Build history of the part. All positions in model axes, mm. Face numbers are marked on the shaded views. A direction names the side the tool comes from. Round coordinates to 2 decimals unless told otherwise and drop trailing zeros. Write each loop counter-clockwise with the first axis right and the second up, starting at its lowest first coordinate (ties: lowest second). Pieces come first, ordered by that corner, then holes.
1) Saw through at A-A (y = 97.5). Write the cut outline in (x, z).
2) Flat gauge pins, fed straight in: pin 1 (1.5 mm diameter, centred on x = 5.5, z = 10.5, fed in from -Y); pin 2 (2 mm diameter, centred on x = -6, y = 47.5, fed in from +Z); pin 3 (6 mm diameter, centred on x = 6, y = 79, fed in from -Z). Where does each tip first touch, or does it go through?
3) Wall check: probe 1 along Y at (x, z) = (3.5, -1.5); probe 2 along Y at (x, z) = (7.25, 1.5); probe 3 along X at (y, z) = (10.5, 7.25). Give the ranges that are in metal, low to high.
4) Pull direction Y, two halves, no side cores. Call the marked faces 3 and 4: +Y half, -Y half, draft (parallel to the pull), parting line (faces both ways), or undercut.
5) Which spindle directions (+Z, -Z, +X, -X, +Y, -Y) get a long thin tool onto all of the face, cutting with end or side? Do the marked faces 1 and 2. Say none if no direction does.
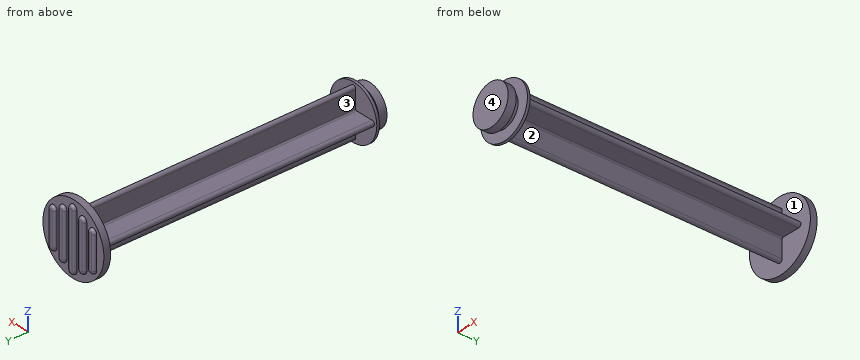
from build123d import *

# Parameters (mm, degrees)
BOSS_EXTRUDE1_DEPTH = 102
SKETCH3_R           = 13
BOSS_EXTRUDE2_DEPTH = 2.5
BOSS_EXTRUDE3_DEPTH = 1
FILLET1_R           = 1


with BuildPart() as part:
    # Sketch1 → Revolve1 (revolve)
    with BuildSketch(Plane.XY, mode=Mode.PRIVATE) as revolve1_sk:
        Polygon((0, 0), (7.5, 0), (7.5, 3), (6, 3), (6, 5), (10, 5), (10, 6), (0, 6), align=None)
    revolve(revolve1_sk.sketch.rotate(Axis((0, 6, 0), (0, -1, 0)), 180), axis=Axis((0, 6, 0), (0, -1, 0)))

    # Sketch2 → Boss-Extrude1 (add)
    with BuildSketch(Plane(origin=(0, 6, 0), x_dir=(1, 0, 0), z_dir=(0, 1, 0))):
        with BuildLine():
            Line((-1, 8), (-1, 1.5))
            ThreePointArc((-1, 1.5), (-1.146446609, 1.146446609), (-1.5, 1))
            Line((-1.5, 1), (-8, 1))
            ThreePointArc((-8, 1), (-9, 0), (-8, -1))
            Line((-8, -1), (-1.5, -1))
            ThreePointArc((-1.5, -1), (-1.146446609, -1.146446609), (-1, -1.5))
            Line((-1, -1.5), (-1, -8))
            ThreePointArc((-1, -8), (0, -9), (1, -8))
            Line((1, -8), (1, -1.5))
            ThreePointArc((1, -1.5), (1.146446609, -1.146446609), (1.5, -1))
            Line((1.5, -1), (8, -1))
            ThreePointArc((8, -1), (9, 0), (8, 1))
            Line((8, 1), (1.5, 1))
            ThreePointArc((1.5, 1), (1.146446609, 1.146446609), (1, 1.5))
            Line((1, 1.5), (1, 8))
            ThreePointArc((1, 8), (0, 9), (-1, 8))
        make_face()
    extrude(amount=BOSS_EXTRUDE1_DEPTH)

    # Sketch3 → Boss-Extrude2 (add)
    with BuildSketch(Plane(origin=(0, 108, 0), x_dir=(1, 0, 0), z_dir=(0, 1, 0))):
        with Locations(Location((0, 0, 0), (0, 0, 180))):
            Circle(SKETCH3_R)
    extrude(amount=BOSS_EXTRUDE2_DEPTH)

    # Sketch4 → Boss-Extrude3 (add)
    with BuildSketch(Plane(origin=(0, 110.5, 0), x_dir=(1, 0, 0), z_dir=(0, 1, 0))):
        with BuildLine():
            Line((-1.5, 10), (-1.5, -10))
            ThreePointArc((-1.5, -10), (0, -11.5), (1.5, -10))
            Line((1.5, -10), (1.5, 10))
            ThreePointArc((1.5, 10), (0, 11.5), (-1.5, 10))
        make_face()
        with BuildLine():
            Line((-5.7, 8), (-5.7, -8))
            ThreePointArc((-5.7, -8), (-4.2, -9.5), (-2.7, -8))
            Line((-2.7, -8), (-2.7, 8))
            ThreePointArc((-2.7, 8), (-4.2, 9.5), (-5.7, 8))
        make_face()
        with BuildLine():
            Line((-9.9, 6), (-9.9, -6))
            ThreePointArc((-9.9, -6), (-8.4, -7.5), (-6.9, -6))
            Line((-6.9, -6), (-6.9, 6))
            ThreePointArc((-6.9, 6), (-8.4, 7.5), (-9.9, 6))
        make_face()
        with BuildLine():
            Line((9.9, 6), (9.9, -6))
            ThreePointArc((9.9, -6), (8.4, -7.5), (6.9, -6))
            Line((6.9, -6), (6.9, 6))
            ThreePointArc((6.9, 6), (8.4, 7.5), (9.9, 6))
        make_face()
        with BuildLine():
            Line((5.7, 8), (5.7, -8))
            ThreePointArc((5.7, -8), (4.2, -9.5), (2.7, -8))
            Line((2.7, -8), (2.7, 8))
            ThreePointArc((2.7, 8), (4.2, 9.5), (5.7, 8))
        make_face()
    extrude(amount=BOSS_EXTRUDE3_DEPTH)

    # Fillet1
    fillet1_edges = [part.edges().sort_by_distance(p)[0] for p in [
        (9.9, 111.5, 0),
        (8.4, 111.5, 7.5),
        (6.9, 111.5, 0),
        (8.4, 111.5, -7.5),
        (5.7, 111.5, 0),
        (4.2, 111.5, 9.5),
        (2.7, 111.5, 0),
        (4.2, 111.5, -9.5),
        (1.5, 111.5, 0),
        (0, 111.5, 11.5),
        (-1.5, 111.5, 0),
        (0, 111.5, -11.5),
        (-2.7, 111.5, 0),
        (-4.2, 111.5, 9.5),
        (-5.7, 111.5, 0),
        (-4.2, 111.5, -9.5),
        (-6.9, 111.5, 0),
        (-8.4, 111.5, 7.5),
        (-9.9, 111.5, 0),
        (-8.4, 111.5, -7.5),
    ]]
    fillet(fillet1_edges, radius=FILLET1_R - 0.0001)  # a hair under: the kernel refuses the full size


solid = part.part
Evaluation:
1. outline: (-8, -1) - (-1.5, -1) arc R0.5 cw to (-1, -1.5) - (-1, -8) arc R1 ccw to (1, -8) - (1, -1.5) arc R0.5 cw to (1.5, -1) - (8, -1) arc R1 ccw to (8, 1) - (1.5, 1) arc R0.5 cw to (1, 1.5) - (1, 8) arc R1 ccw to (-1, 8) - (-1, 1.5) arc R0.5 cw to (-1.5, 1) - (-8, 1) arc R1 ccw to start
2. pin 1: stops at y = 108
2. pin 2: stops at z = 1
2. pin 3: stops at z = -1
3. probe 1: y = 0 to 6, 108 to 111.48
3. probe 2: y = 0 to 3, 5 to 6, 108 to 111.26
3. probe 3: x = -1 to 1
4. face 3: undercut
4. face 4: -Y half
5. face 1: none
5. face 2: -Z, +X
